For this review, use the dimensioned drawing (mm, ordinates from the lowest corner) and the shaded views. Coordinates: 2 decimals unless noted, no trailing zeros. Order: outer loops, then holes, each group sorted by start corner. A loop starts at its lowest first (then second) coordinate and runs counter-clockwise, first axis right, second up. Notation, with made-up numbers: M -2.75,85.5 L 21.25,85.5 A31 ccw 21.25,116.5 Z; hole C -5,-14 d1. An arc over 180 degrees is marked long. Write each question's results on one line, items separated by ' | '.
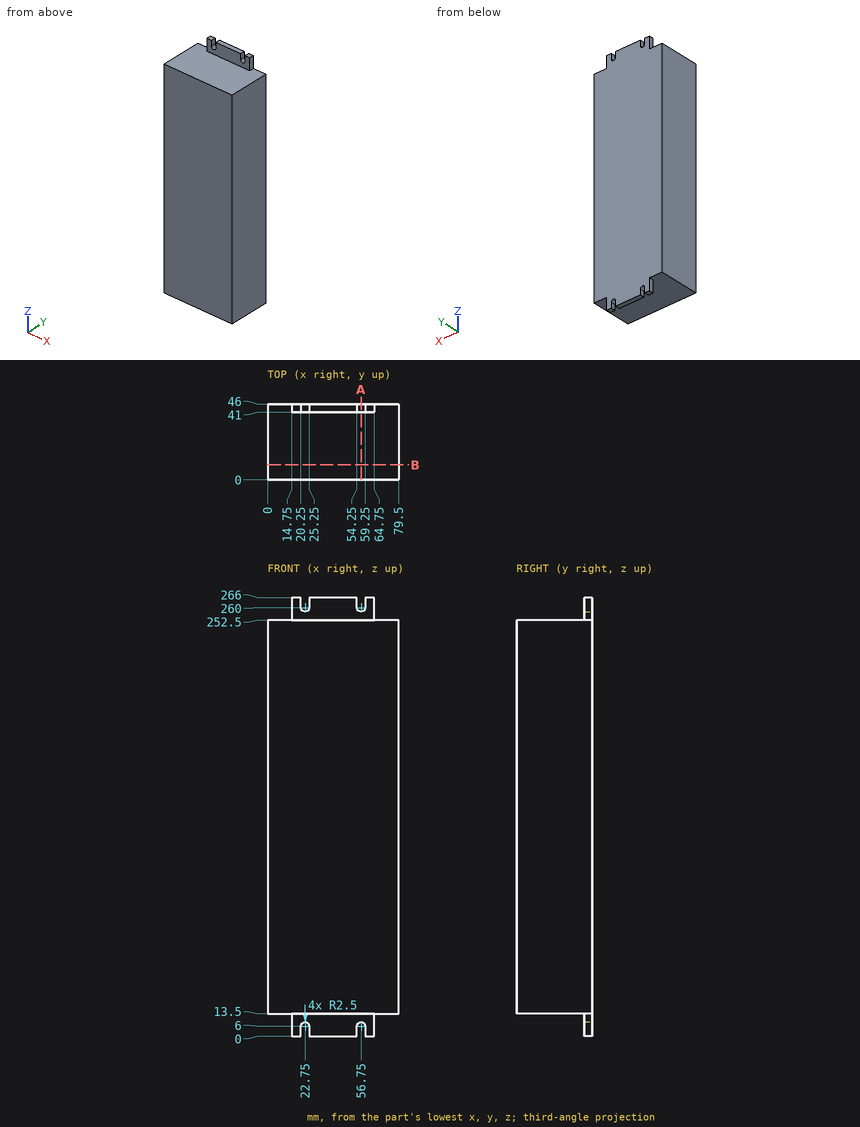
1) Take a section at A-A on x = 56.75. State the section outline as (y, z) points.
Solutions:
outline: M 0,13.5 L 41,13.5 L 41,8.5 L 46,8.5 L 46,257.5 L 41,257.5 L 41,252.5 L 0,252.5 Z
2) Take a section at B-B on y = 9. State the section outline as (x, z) points.
Solutions:
outline: M 0,13.5 L 79.5,13.5 L 79.5,252.5 L 0,252.5 Z
3) To check wall thickness, follow line 1 along Y through (x, z) = (24.5, 11); line 2 along Z through (x, y) = (61, 22.5). State the ranges of each line that lie inside material, in increasing order.
Solutions:
line 1: 41 to 46 | line 2: 13.5 to 252.5
4) For pin 1 (5.5 mm diameter, centred on y = 44, z = 256.5, fed in from +X); pin 2 (5.5 mm diameter, centred on y = 43.5, z = 263, fed in from -X); pin 3 (11 mm diameter, centred on x = 34, z = 259.5, fed in from -Y), all flat-tipped, find the tip position at first contact; note any pin that passes through.
Solutions:
pin 1: x = 64.75 | pin 2: x = 14.75 | pin 3: y = 41
